```python
from build123d import *

# Parameters (mm, degrees)
SKETCH1_R           = 30
BOSS_EXTRUDE1_DEPTH = 4
SKETCH2_R           = 6
BOSS_EXTRUDE2_DEPTH = 6
CUT_EXTRUDE1_DEPTH  = 44.588989435
SKETCH4_R           = 1.4
CUT_EXTRUDE2_DEPTH  = 5
CUT_EXTRUDE3_DEPTH  = 44.588989458


with BuildPart() as part:
    # Sketch1 → Boss-Extrude1 (new body)
    with BuildSketch(Plane(origin=(0, 0, 0), x_dir=(1, 0, 0), z_dir=(0, 1, 0))):
        with Locations(Location((0, 0, 0), (0, 0, 270))):
            Circle(SKETCH1_R)
    extrude(amount=BOSS_EXTRUDE1_DEPTH)

    # Sketch2 → Boss-Extrude2 (add)
    with BuildSketch(Plane(origin=(0, 4, 0), x_dir=(1, 0, 0), z_dir=(0, 1, 0))):
        with Locations(Location((0, 0, 0), (0, 0, 270))):
            Circle(SKETCH2_R)
    extrude(amount=BOSS_EXTRUDE2_DEPTH)

    # Sketch3 → Cut-Extrude1 (cut, through all)
    with BuildSketch(Plane(origin=(0, 10, 0), x_dir=(1, 0, 0), z_dir=(0, 1, 0))):
        with BuildLine():
            Line((2.121320344, -1.75), (2.121320344, 1.75))
            ThreePointArc((2.121320344, 1.75), (-2.75, 0), (2.121320344, -1.75))
        make_face()
    extrude(amount=-CUT_EXTRUDE1_DEPTH, mode=Mode.SUBTRACT)

    # Sketch4 → Cut-Extrude2 (cut)
    with BuildSketch(Plane.ZY.offset(-2.121320344)):
        with Locations((0, 7)):
            Circle(SKETCH4_R)
    extrude(amount=-CUT_EXTRUDE2_DEPTH, mode=Mode.SUBTRACT)

    # Sketch5 → Cut-Extrude3 (cut, through all)
    with BuildSketch(Plane(origin=(0, 0, 0), x_dir=(-1, 0, 0), z_dir=(0, -1, 0))):
        with BuildLine():
            ThreePointArc((1.5, -26.958301133), (19.091883092, -19.091883092), (26.958301133, -1.5))
            Line((26.958301133, -1.5), (5.809475019, -1.5))
            ThreePointArc((5.809475019, -1.5), (4.242640687, -4.242640687), (1.5, -5.809475019))
            Line((1.5, -5.809475019), (1.5, -26.958301133))
        make_face()
        with BuildLine():
            ThreePointArc((-26.958301133, -1.5), (-19.091883092, -19.091883092), (-1.5, -26.958301133))
            Line((-1.5, -26.958301133), (-1.5, -5.809475019))
            ThreePointArc((-1.5, -5.809475019), (-4.242640687, -4.242640687), (-5.809475019, -1.5))
            Line((-5.809475019, -1.5), (-26.958301133, -1.5))
        make_face()
        with BuildLine():
            Line((-1.5, 5.809475019), (-1.5, 26.958301133))
            ThreePointArc((-1.5, 26.958301133), (-19.091883092, 19.091883092), (-26.958301133, 1.5))
            Line((-26.958301133, 1.5), (-5.809475019, 1.5))
            ThreePointArc((-5.809475019, 1.5), (-4.242640687, 4.242640687), (-1.5, 5.809475019))
        make_face()
        with BuildLine():
            Line((5.809475019, 1.5), (26.958301133, 1.5))
            ThreePointArc((26.958301133, 1.5), (19.091883092, 19.091883092), (1.5, 26.958301133))
            Line((1.5, 26.958301133), (1.5, 5.809475019))
            ThreePointArc((1.5, 5.809475019), (4.242640687, 4.242640687), (5.809475019, 1.5))
        make_face()
    extrude(amount=-CUT_EXTRUDE3_DEPTH, mode=Mode.SUBTRACT)


solid = part.part
```
Work out the finished part from the listing and answer in its coordinate system (mm). A direction names the side the tool comes from. Coordinates: 2 decimals unless noted, no trailing zeros. Loops run counter-clockwise (first coordinate to the right, second up) from the corner with the lowest first, then second, coordinate; pieces in that order, holes last. Notation, with made-up numbers: M 2,-22 L 57,-22 A15 cw 57,1 Z; hole C 88.5,-37 d8. An arc over 180 degrees is marked long. Use CSV: the item, a comma, the result in double quotes. Start each with the question number.
(1) For a pull along Z with two mould halves and no side action, classify faces 4 (the face through (-17, 2, 1.5)), 5 (the face through (-19.286, 1.972, -18.896)), 6 (the face through (0.4, 4, 6.2)), 7 (the face through (1.32, 1.97, -29.97)) as +Z half, -Z half, draft (parallel to the pull), parting line (faces both ways), or undercut.
(2) Consider line 1 (X direction, y = 4.5, z = 0); line 2 (X direction, y = 2, z = 16); line 3 (Z direction, x = 2, y = 0.5). Determine where each line is inside the solid, lowest interval first.
(3) Find section A-A, the plane z = 0. Give the vertices of the cut face in (x, y).
(4) Find section D-D, the plane x = 19. Give the vertices of the cut face in (y, z), then the cut area to 3 significant figures.
(5) For faces 1 (the face through (-1, 10, 3)), 2 (the face through (18.896, 1.972, -19.286)), 3 (the face through (4.036, 5.633, -0.303)), determine the directions among +Z, -Z, +X, -X, +Y, -Y from which every point of the face is accessible in a straight line to the end or side of a thin tool.
(6) Find section B-B, the plane y = 0.75. Give the vertices of the cut face in (x, z), then the cut area to 3 significant figures.
(7) Find section C-C, the plane x = 0. Give the vertices of the cut face in (y, z), then the cut area to 3 significant figures.
(8) Given pin 1 Ø6 at (x, y) = (-11, 1) entering from +Z; pin 2 Ø1.2 at (x, y) = (-16, 2) entering from +Z; pin 3 Ø3 at (y, z) = (3, -20.5) entering from +X, each flat-ended and moving along its own axis, determine where each tip first touches the part or whether it passes through.
Recorded:
1,face 4,"undercut"
1,face 5,"undercut"
1,face 6,"draft"
1,face 7,"parting line"
2,line 1,"x = -6 to -2.75, 2.12 to 6"
2,line 2,"x = -25.38 to -21.75, -1.5 to 1.5, 21.75 to 25.38"
2,line 3,"z = -29.93 to -26.93, -5.66 to -1.89, 1.89 to 5.66, 26.93 to 29.93"
3,outline,"M -30,0 L -2.75,0 L -2.75,10 L -6,10 L -6,4 L -30,4 Z; M 2.12,0 L 30,0 L 30,4 L 6,4 L 6,5.6 L 2.12,5.6 Z; M 2.12,8.4 L 6,8.4 L 6,10 L 2.12,10 Z"
4,outline,"M 0,-23.22 L 4,-23.22 L 4,-19.18 L 0,-19.18 Z; M 0,-1.5 L 4,-1.5 L 4,1.5 L 0,1.5 Z; M 0,19.18 L 4,19.18 L 4,23.22 L 0,23.22 Z"
4,area,"44.3 mm^2"
5,face 1,"+Z, -Z, +X, -X, +Y"
5,face 2,"+Y, -Y"
5,face 3,"+X"
6,outline,"C 0,0 d60; hole M -26.96,-1.5 A27 ccw -1.5,-26.96 L -1.5,-5.81 A6 cw -5.81,-1.5 Z; hole M -26.96,1.5 L -5.81,1.5 A6 cw -1.5,5.81 L -1.5,26.96 A27 ccw Z; hole M 1.5,-26.96 A27 ccw 26.96,-1.5 L 5.81,-1.5 A6 cw 1.5,-5.81 Z; hole M 1.5,5.81 A6 cw 5.81,1.5 L 26.96,1.5 A27 ccw 1.5,26.96 Z; hole M 2.12,-1.75 L 2.12,1.75 A2.75 ccw long Z"
6,area,"881 mm^2"
7,outline,"M 0,-30 L 4,-30 L 4,-6 L 10,-6 L 10,-2.75 L 0,-2.75 Z; M 0,2.75 L 10,2.75 L 10,6 L 4,6 L 4,30 L 0,30 Z"
7,area,"257 mm^2"
8,pin 1,"stops at z = 28.91"
8,pin 2,"stops at z = 25.75"
8,pin 3,"stops at x = 23.22"
